The listing builds one solid part. Answer for the finished solid, in the listing's coordinates (mm). Face numbers are marked on the shaded views. A direction names the side the tool comes from. Coordinates: 2 decimals unless noted, no trailing zeros. Write each loop counter-clockwise with the first axis right and the second up, starting at its lowest first coordinate (ties: lowest second). Pieces come first, ordered by that corner, then holes. Notation, with made-up numbers: M 63.5,-13.5 L 112.5,-13.5 A22 ccw 112.5,8.5 Z; hole C 25.25,12.25 d5. An arc over 180 degrees is marked long. Answer as CSV lines item,"result".
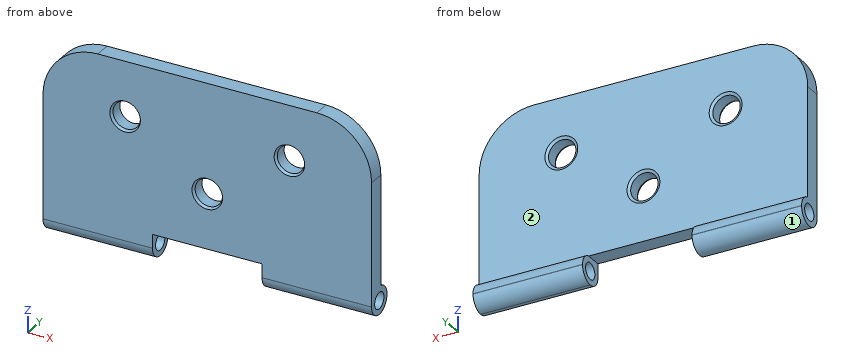
```python
from build123d import *
from OCP.BRepFilletAPI import BRepFilletAPI_MakeChamfer

# Parameters (mm, degrees)
SZKIC1_W                    = 60
SZKIC1_H                    = 30
DODANIE_WYCI_GNI_CIE1_DEPTH = 3
SZKIC2_R                    = 2.5
WYTNIJ_WYCI_GNI_CIE1_DEPTH  = 5
SZKIC4_W                    = 20
SZKIC4_H                    = 3
DODANIE_WYCI_GNI_CIE2_DEPTH = 5
SZKIC5_W                    = 20
SZKIC5_H                    = 5
DODANIE_WYCI_GNI_CIE3_DEPTH = 2
ZAOKR_GLENIE1_R             = 2.5
SZKIC6_R                    = 1.5
WYTNIJ_WYCI_GNI_CIE2_DEPTH  = 60
ZAOKR_GLENIE2_R             = 10
SFAZOWANIE1_SIZE            = 0.5
SFAZOWANIE1_SIZE2           = 0.288675135


with BuildPart() as part:
    # Szkic1 → Dodanie-wyciągnięcie1 (new body)
    with BuildSketch(Plane(origin=(0, 0, 0), x_dir=(1, 0, 0), z_dir=(0, 1, 0))):
        Rectangle(SZKIC1_W, SZKIC1_H)
    extrude(amount=DODANIE_WYCI_GNI_CIE1_DEPTH)

    # Szkic2 → Wytnij-wyciągnięcie1 (cut)
    with BuildSketch(Plane(origin=(0, 3, 0), x_dir=(1, 0, 0), z_dir=(0, 1, 0))):
        with Locations(Location((-15, -5, 0), (0, 0, 270))):
            Circle(SZKIC2_R)
        with Locations(Location((15, -5, 0), (0, 0, 270))):
            Circle(SZKIC2_R)
        with Locations(Location((0, 5, 0), (0, 0, 270))):
            Circle(SZKIC2_R)
    extrude(amount=-WYTNIJ_WYCI_GNI_CIE1_DEPTH, mode=Mode.SUBTRACT)

    # Szkic4 → Dodanie-wyciągnięcie2 (add)
    with BuildSketch(Plane(origin=(0, 0, -15), x_dir=(-1, 0, 0), z_dir=(0, 0, -1))):
        with Locations((-20, 1.5)):
            Rectangle(SZKIC4_W, SZKIC4_H)
        with Locations((20, 1.5)):
            Rectangle(SZKIC4_W, SZKIC4_H)
    extrude(amount=DODANIE_WYCI_GNI_CIE2_DEPTH)

    # Szkic5 → Dodanie-wyciągnięcie3 (add)
    with BuildSketch(Plane(origin=(0, 3, 0), x_dir=(1, 0, 0), z_dir=(0, 1, 0))):
        with Locations((-20, 17.5)):
            Rectangle(SZKIC5_W, SZKIC5_H)
        with Locations((20, 17.5)):
            Rectangle(SZKIC5_W, SZKIC5_H)
    extrude(amount=DODANIE_WYCI_GNI_CIE3_DEPTH)

    # Zaokrąglenie1
    # the kernel refuses this fillet: 2.5 mm, written as the material it takes off along each edge
    with BuildSketch(Plane(origin=(-36.25, 0, -20), x_dir=(0, 1, 0), z_dir=(1, 0, 0)), Plane(origin=(-36.25, 5, -20), x_dir=(0, 0, 1), z_dir=(1, 0, 0)), Plane(origin=(3.75, 5, -20), x_dir=(0, 0, 1), z_dir=(1, 0, 0))) as zaokr_glenie1_piece_1:
        with BuildLine():
            CenterArc((ZAOKR_GLENIE1_R, ZAOKR_GLENIE1_R), ZAOKR_GLENIE1_R, 180, 90)
            Line((0, ZAOKR_GLENIE1_R), (-ZAOKR_GLENIE1_R * 0.02, ZAOKR_GLENIE1_R))
            Line((-ZAOKR_GLENIE1_R * 0.02, ZAOKR_GLENIE1_R), (-ZAOKR_GLENIE1_R * 0.02, -ZAOKR_GLENIE1_R * 0.02))
            Line((-ZAOKR_GLENIE1_R * 0.02, -ZAOKR_GLENIE1_R * 0.02), (ZAOKR_GLENIE1_R, -ZAOKR_GLENIE1_R * 0.02))
            Line((ZAOKR_GLENIE1_R, -ZAOKR_GLENIE1_R * 0.02), (ZAOKR_GLENIE1_R, 0))
        make_face()
    extrude(amount=32.5, mode=Mode.SUBTRACT)
    with BuildSketch(Plane(origin=(-3.876275643, 5, -15), x_dir=(0, -1.0, -1.666222715356868e-12), z_dir=(-1, 0, 0)), Plane(origin=(36.123724357, 5, -15), x_dir=(0, -1.0, -1.666222715356868e-12), z_dir=(-1, 0, 0))) as zaokr_glenie1_piece_2:
        with BuildLine():
            CenterArc((2.5, -2.449489743), ZAOKR_GLENIE1_R, 101.536959033, 78.463040967)
            Line((0, -2.449489743), (-0.05, -2.449489743))
            Line((-0.05, -2.449489743), (-0.05, 0))
            Line((-0.05, 0), (0, 0.05))
            ThreePointArc((0, 0.05), (1, 0.05), (1.99, 0.048989795))
            Line((1.99, 0.048989795), (2, 0))
        make_face()
    extrude(amount=32.247448714, mode=Mode.SUBTRACT)
    with BuildSketch(Plane(origin=(36.25, 0, -20), x_dir=(0, 1, 0), z_dir=(-1, 0, 0))) as zaokr_glenie1_piece_3:
        with BuildLine():
            CenterArc((ZAOKR_GLENIE1_R, -ZAOKR_GLENIE1_R), ZAOKR_GLENIE1_R, 90, 90)
            Line((0, -ZAOKR_GLENIE1_R), (-ZAOKR_GLENIE1_R * 0.02, -ZAOKR_GLENIE1_R))
            Line((-ZAOKR_GLENIE1_R * 0.02, -ZAOKR_GLENIE1_R), (-ZAOKR_GLENIE1_R * 0.02, ZAOKR_GLENIE1_R * 0.02))
            Line((-ZAOKR_GLENIE1_R * 0.02, ZAOKR_GLENIE1_R * 0.02), (ZAOKR_GLENIE1_R, ZAOKR_GLENIE1_R * 0.02))
            Line((ZAOKR_GLENIE1_R, ZAOKR_GLENIE1_R * 0.02), (ZAOKR_GLENIE1_R, 0))
        make_face()
    extrude(amount=32.5, mode=Mode.SUBTRACT)

    # Szkic6 → Wytnij-wyciągnięcie2 (cut)
    with BuildSketch(Plane(origin=(30, 0, 0), x_dir=(0, 0, -1), z_dir=(1, 0, 0))):
        with Locations((17.5, 2.5)):
            Circle(SZKIC6_R)
    extrude(amount=-WYTNIJ_WYCI_GNI_CIE2_DEPTH, mode=Mode.SUBTRACT)

    # Zaokrąglenie2
    zaokr_glenie2_edges = [part.edges().sort_by_distance(p)[0] for p in [
        (30, 1.5, 15),
        (-30, 1.5, 15),
    ]]
    fillet(zaokr_glenie2_edges, radius=ZAOKR_GLENIE2_R)

    # Sfazowanie1: one chamfer whose edges measure the first distance from different faces: ONE call of the kernel's chamfer builder (chamfer() names one face for all edges)
    sfazowanie1_edges_1 = [part.edges().sort_by_distance(p)[0] for p in [
        (-15, 0, 2.5),
    ]]
    sfazowanie1_side_1 = [part.faces().sort_by_distance(p)[0] for p in [
        (-15, 1.5, 2.5),
    ]]
    sfazowanie1_edges_2 = [part.edges().sort_by_distance(p)[0] for p in [
        (-15, 3, 2.5),
        (15, 3, 2.5),
        (0, 3, -7.5),
    ]]
    sfazowanie1_side_2 = [part.faces().sort_by_distance(p)[0] for p in [
        (0, 3, -0.380473171),
    ]]
    sfazowanie1_edges_3 = [part.edges().sort_by_distance(p)[0] for p in [
        (15, 0, 2.5),
    ]]
    sfazowanie1_side_3 = [part.faces().sort_by_distance(p)[0] for p in [
        (15, 1.5, 2.5),
    ]]
    sfazowanie1_edges_4 = [part.edges().sort_by_distance(p)[0] for p in [
        (0, 0, -7.5),
    ]]
    sfazowanie1_side_4 = [part.faces().sort_by_distance(p)[0] for p in [
        (0, 1.5, -7.5),
    ]]
    sfazowanie1 = BRepFilletAPI_MakeChamfer(part.part.solid().wrapped)
    for e in sfazowanie1_edges_1:
        sfazowanie1.Add(SFAZOWANIE1_SIZE, SFAZOWANIE1_SIZE2, e.wrapped, sfazowanie1_side_1[0].wrapped)  # the first distance lies on this face
    for e in sfazowanie1_edges_2:
        sfazowanie1.Add(SFAZOWANIE1_SIZE, SFAZOWANIE1_SIZE2, e.wrapped, sfazowanie1_side_2[0].wrapped)  # the first distance lies on this face
    for e in sfazowanie1_edges_3:
        sfazowanie1.Add(SFAZOWANIE1_SIZE, SFAZOWANIE1_SIZE2, e.wrapped, sfazowanie1_side_3[0].wrapped)  # the first distance lies on this face
    for e in sfazowanie1_edges_4:
        sfazowanie1.Add(SFAZOWANIE1_SIZE, SFAZOWANIE1_SIZE2, e.wrapped, sfazowanie1_side_4[0].wrapped)  # the first distance lies on this face
    add(Compound.cast(sfazowanie1.Shape()), mode=Mode.REPLACE)


solid = part.part
```
Q1. Find section A-A (x = -15). Give the vertices of the cut face in (y, z), and give its area (3 significant figures).
Output:
outline,"M 0,-17.5 A2.5 ccw 5,-17.5 L 5,-17.45 A2.5 ccw 3,-15 L 3,2 L 2.71,2.5 L 0.5,2.5 L 0,2.21 Z; M 0,7.79 L 0.5,7.5 L 2.71,7.5 L 3,8 L 3,15 L 0,15 Z; hole C 2.5,-17.5 d3"
area,"88.7 mm2"
Q2. For the marked faces 1 and 2, determine the directions among +Z, -Z, +X, -X, +Y, -Y from which every point of the face is accessible in a straight line to the end or side of a thin tool.
Output:
face 1,"-Z, +X, -X"
face 2,"+Z, +X, -X, +Y"
Q3. Find section C-C (x = 0). Give the vertices of the cut face in (y, z), and give its area (3 significant figures).
Output:
outline,"M 0,-15 L 3,-15 L 3,-8 L 2.71,-7.5 L 0.5,-7.5 L 0,-7.79 Z; M 0,-2.21 L 0.5,-2.5 L 2.71,-2.5 L 3,-2 L 3,15 L 0,15 Z"
area,"74.7 mm2"
Q4. Find section B-B (z = -5). Give the vertices of the cut face in (x, y), and give its area (3 significant figures).
Output:
outline,"M -30,0 L -2.79,0 L -2.5,0.5 L -2.5,2.71 L -3,3 L -30,3 Z; M 2.5,0.5 L 2.79,0 L 30,0 L 30,3 L 3,3 L 2.5,2.71 Z"
area,"165 mm2"
Q5. Flat-ended cylindrical pins translate along their axes: pin 1 Ø1.5 at (x, y) = (-2.5, 1) entering from -Z; pin 2 Ø1 at (x, z) = (5, -2.5) entering from +Y; pin 3 Ø4.5 at (x, z) = (-15, 5) entering from -Y. Find the tip coordinate at first contact, or state that the pin passes through.
Output:
pin 1,"z = -15"
pin 2,"y = 3"
pin 3,"through"
Q6. Find section D-D (z = 3.5). Count the separate pieces of the cut face and the enclosed holes in it, and give its area (3 significant figures).
Output:
separate pieces,"3"
enclosed holes,"0"
area,"155 mm2"
Q7. Straight lines are drawn through the part: line 1 (X direction, y = 4.15, z = -17); line 2 (Y direction, x = -8.5, z = -4); line 3 (Y direction, x = 16, z = -17). For each, find the intervals that lie inside material, in ascending order.
Output:
line 1,"-30 to -10, 10 to 30"
line 2,"0 to 3"
line 3,"0 to 1.09, 3.91 to 4.96"
